Autodesk Inventor part; units mm, degrees
ref_plane "YZ Plane" through (0, 0, 0) normal (1, 0, 0) x (0, 1, 0)
ref_plane "XZ Plane" through (0, 0, 0) normal (0, 1, 0) x (-1, 0, 0)
ref_plane "XY Plane" through (0, 0, 0) normal (0, 0, 1) x (1, 0, 0)
sketch "Sketch1" plane through (0, 0, 0) normal (0, 0, 1) x (1, 0, 0)
  line L0 (0, 5.785) -> (-2.44, 5.785)
  line L1 (-2.44, 5.785) -> (-2.44, 3.785)
  line L2 (-2.44, 3.785) -> (-5.055, 3.785)
  line L3 (-5.055, 3.785) -> (-5.055, -4.575)
  line L4 (-5.055, -4.575) -> (-3.26, -4.575)
  line L5 (-3.26, -4.575) -> (-3.26, -5.785)
  line L6 (-3.26, -5.785) -> (0, -5.785)
  line L7 (0, -5.785) -> (0, 5.785)
  point P0 (0, 0)
  point P1 (0, 0)
  dimension "d0" = 11.57
  dimension "d1" = 10.11
  dimension "d2" = 4.88
  dimension "d3" = 6.52
  dimension "d4" = 2
  dimension "d5" = 1.21
revolve "Revolution1" add sketch "Sketch1" angle 360 about axis through (0, -5.785, 0) along (0, 1, 0)
fillet "Fillet1" radius 1.75 2 edges at (5.055, 3.785, 0) (5.055, -4.575, 0)
fillet "Fillet2" radius 0.4 1 edges at (2.44, 5.785, 0)
sketch "Sketch2" plane through (0, -5.785, 0) normal (0, -1, 0) x (1, 0, 0)
  circle A0 centre (0, 0) radius 3.26
  circle A1 centre (0, 0) radius 2.5
  dimension "d9" = 5
extrude "Extrusion1" cut sketch "Sketch2" against normal blind 3 contours A1
properties part number "HEAD" material "250"
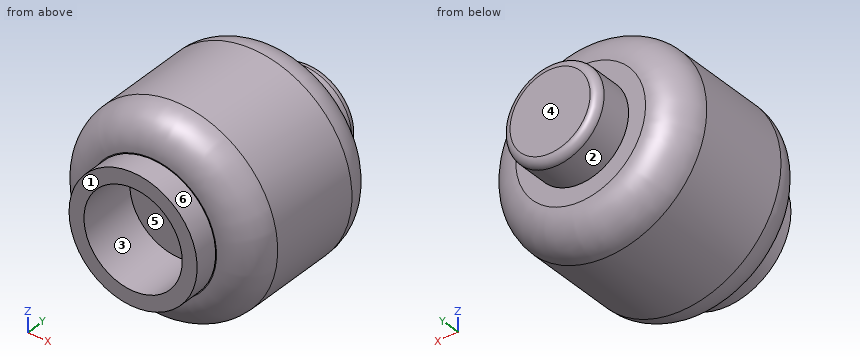
Work out the finished part from the listing and answer in its coordinate system (mm). Face numbers are marked on the shaded views. A direction names the side the tool comes from. Give positions to 0.01 mm unless a question says otherwise; leave off trailing zeros. Order: outer loops, then holes, each group sorted by start corner. A loop starts at its lowest first (then second) coordinate and runs counter-clockwise, first axis right, second up. Notation, with made-up numbers: M 79.25,52.5 L 127.25,52.5 A24 ccw 127.25,78.5 Z; hole C 32,49 d6. An arc over 180 degrees is marked long. Return JSON: item names as keys, results as strings.
Q1. Each of these flat-tipped pins is pushed along its axis until it touches: pin 1 (1.5 mm diameter, centred on x = -2.5, z = -1, fed in from +Y) (3 decimals); pin 2 (5 mm diameter, centred on y = 4, z = 4, fed in from -X); pin 3 (4 mm diameter, centred on x = -2.5, y = -2.5, fed in from -Z); pin 4 (1 mm diameter, centred on y = -4.5, z = -2, fed in from -X). Where does it stop, or does it pass through?
Answer below:
{"pin 1": "stops at y = 5.785", "pin 2": "stops at x = -4.57", "pin 3": "stops at z = -5.03", "pin 4": "stops at x = -4.19"}
Q2. Find the intervals of material crossed by line 1 along Y through (x, z) = (-1, 1.5) (3 decimals); line 2 along Z through (x, y) = (0, -4.95); line 3 along Y through (x, z) = (3.25, -1), in increasing order. Write a range as [from, to].
Answer below:
{"line 1": "y = [-2.785, 5.785]", "line 2": "z = [-3.26, -2.5], [2.5, 3.26]", "line 3": "y = [-4.57, 3.78]"}
Q3. The mould has two halves that part along Z. Classify the marked faces 3, 4, 5 and 6: pulls with the +Z half, pulls with the -Z half, needs draft (parallel to the pull), parting line crosses it, or undercut.
Answer below:
{"face 3": "undercut", "face 4": "needs draft", "face 5": "undercut", "face 6": "parting line crosses it"}
Q4. Find section C-C, the plane y = -2. Write down the section's boundary in (x, z) (3 decimals).
Answer below:
{"outline": "C 0,0 d10.11"}
Q5. Find section A-A, the plane x = 0. Write down the section's boundary in (y, z) (3 decimals), and give its area (3 significant figures).
Answer below:
{"outline": "M -5.785,-3.26 L -4.575,-3.26 L -4.575,-3.305 A1.75 ccw -2.825,-5.055 L 2.035,-5.055 A1.75 ccw 3.785,-3.305 L 3.785,-2.44 L 5.385,-2.44 A0.4 ccw 5.785,-2.04 L 5.785,2.04 A0.4 ccw 5.385,2.44 L 3.785,2.44 L 3.785,3.305 A1.75 ccw 2.035,5.055 L -2.825,5.055 A1.75 ccw -4.575,3.305 L -4.575,3.26 L -5.785,3.26 L -5.785,2.5 L -2.785,2.5 L -2.785,-2.5 L -5.785,-2.5 Z", "area": "84.5 mm^2"}
Q6. Which of the six approach directions +Z, -Z, +X, -X, +Y, -Y give full straight-line access (tool end or side, diameter ignored) to the marked faces 1 and 2?
Answer below:
{"face 1": "+Z, -Z, +X, -X, -Y", "face 2": "+Y"}
Q7. Find section B-B, the plane z = 0. Write down the section's boundary in (x, y) (3 decimals).
Answer below:
{"outline": "M -5.055,-2.825 A1.75 ccw -3.305,-4.575 L -3.26,-4.575 L -3.26,-5.785 L -2.5,-5.785 L -2.5,-2.785 L 2.5,-2.785 L 2.5,-5.785 L 3.26,-5.785 L 3.26,-4.575 L 3.305,-4.575 A1.75 ccw 5.055,-2.825 L 5.055,2.035 A1.75 ccw 3.305,3.785 L 2.44,3.785 L 2.44,5.385 A0.4 ccw 2.04,5.785 L -2.04,5.785 A0.4 ccw -2.44,5.385 L -2.44,3.785 L -3.305,3.785 A1.75 ccw -5.055,2.035 Z"}
Q8. Find section D-D, the plane y = -4. Write down the section's boundary in (x, z), and give its area (3 significant figures).
Answer below:
{"outline": "C 0,0 d9.2; hole C 0,0 d5", "area": "46.9 mm^2"}
